from build123d import *

# Parameters (mm, degrees)
SKETCH_1_W          = 6.5
SKETCH_1_H          = 35
EXTRUDE_1_DEPTH     = 6
SKETCH_2_W          = 2.5
SKETCH_2_H          = 2.967804408
CUT_EXTRUDE_1_DEPTH = 61
SKETCH_3_W          = 6.5
SKETCH_3_H          = 15
EXTRUDE_2_DEPTH     = 4.5
SKETCH_4_W          = 6.5
SKETCH_4_H          = 1
CUT_EXTRUDE_2_DEPTH = 503.5
SKETCH_5_W          = 6.5
SKETCH_5_H          = 2
EXTRUDE_3_DEPTH     = 11.5
SKETCH_6_W          = 6.5
SKETCH_6_H          = 2
EXTRUDE_4_DEPTH     = 11.5
SKETCH_7_W          = 3.5
SKETCH_7_H          = 2.5
CUT_EXTRUDE_3_DEPTH = 90.5


with BuildPart() as part:
    # Эскиз1 → Бобышка-Вытянуть1 (new body)
    with BuildSketch(Plane(origin=(0, 0, 0), x_dir=(1, 0, 0), z_dir=(0, 1, 0))):
        with Locations((-18.856267111, 10.244186047)):
            Rectangle(SKETCH_1_W, SKETCH_1_H)
    extrude(amount=EXTRUDE_1_DEPTH)

    # Эскиз2 → Вырез-Вытянуть1 (cut)
    with BuildSketch(Plane.XY.offset(7.255813953)):
        with Locations((-18.856267111, 1.483902204)):
            Rectangle(SKETCH_2_W, SKETCH_2_H)
    extrude(amount=-CUT_EXTRUDE_1_DEPTH, mode=Mode.SUBTRACT)

    # Эскиз3 → Бобышка-Вытянуть2 (add)
    with BuildSketch(Plane(origin=(0, 6, 0), x_dir=(1, 0, 0), z_dir=(0, 1, 0))):
        with Locations((-18.856267111, 10.244186047)):
            Rectangle(SKETCH_3_W, SKETCH_3_H)
    extrude(amount=EXTRUDE_2_DEPTH)

    # Эскиз4 → Вырез-Вытянуть2 (cut)
    with BuildSketch(Plane.XY.offset(7.255813953)):
        with Locations((-18.856267111, 0.5)):
            Rectangle(SKETCH_4_W, SKETCH_4_H)
    extrude(amount=-CUT_EXTRUDE_2_DEPTH, mode=Mode.SUBTRACT)

    # Эскиз5 → Бобышка-Вытянуть3 (add)
    with BuildSketch(Plane(origin=(0, 6, 0), x_dir=(1, 0, 0), z_dir=(0, 1, 0))):
        with Locations((-18.856267111, 18.744186047)):
            Rectangle(SKETCH_5_W, SKETCH_5_H)
    extrude(amount=EXTRUDE_3_DEPTH)

    # Эскиз6 → Бобышка-Вытянуть4 (add)
    with BuildSketch(Plane(origin=(0, 6, 0), x_dir=(1, 0, 0), z_dir=(0, 1, 0))):
        with Locations((-18.856267111, 1.744186047)):
            Rectangle(SKETCH_6_W, SKETCH_6_H)
    extrude(amount=EXTRUDE_4_DEPTH)

    # Эскиз7 → Вырез-Вытянуть3 (cut)
    with BuildSketch(Plane.XY.offset(7.255813953)):
        with Locations((-18.856267111, 2.25)):
            Rectangle(SKETCH_7_W, SKETCH_7_H)
    extrude(amount=-CUT_EXTRUDE_3_DEPTH, mode=Mode.SUBTRACT)


solid = part.part
Geometry: final body of the model. Coordinates: model frame, mm. A direction names the side the tool comes from. Give positions to 0.01 mm unless a question says otherwise; leave off trailing zeros. Write each loop counter-clockwise with the first axis right and the second up, starting at its lowest first coordinate (ties: lowest second). Pieces come first, ordered by that corner, then holes. Notation, with made-up numbers: (64, 8.25) -> (86, 8.25) arc R26 cw to (86, 35.25) -> close; hole circle Ø6 at (53.25, -30). An arc over 180 degrees is marked (long way). Answer as a JSON object with one key per item and string values.
1. Cut plane D-D on y = 6.75. Output: boundary loops of the cut face in (x, z), and give its area (4 significant figures).
Ans:
{"outline": "(-22.11, -19.74) -> (-15.61, -19.74) -> (-15.61, -0.74) -> (-22.11, -0.74) -> close", "area": "123.5 mm^2"}
2. Cut plane C-C on z = 3. Output: boundary loops of the cut face in (x, y), and give its area (4 significant figures).
Ans:
{"outline": "(-22.11, 1) -> (-20.61, 1) -> (-20.61, 3.5) -> (-17.11, 3.5) -> (-17.11, 1) -> (-15.61, 1) -> (-15.61, 6) -> (-22.11, 6) -> close", "area": "23.75 mm^2"}
3. Access query for faces 1 (the flat face through (-20.606, 2, -10)), 2 (the flat face through (-19, 6, -24)), 3 (the flat face through (-19, 6, 3)). Directions: +Z, -Z, +X, -X, +Y, -Y. A direction counts if a zero-diameter tool reaches every point of the face in a straight line with its end or side. Return the directions, or none.
Ans:
{"face 1": "+Z, -Z, -Y", "face 2": "-Z, +X, -X, +Y", "face 3": "+Z, +X, -X, +Y"}
4. Mould query, pull axis Z, two halves, no side actions, for faces 4 (the flat face through (-19, 12, -0.744)), 5 (the flat face through (-19, 17.5, -19)), 6 (the flat face through (-19, 10.5, -10)), 7 (the flat face through (-19, 14, -2.744)). Classes: pulls with the +Z half, pulls with the -Z half, needs draft (parallel to the pull), parting line crosses it, or undercut.
Ans:
{"face 4": "pulls with the +Z half", "face 5": "needs draft", "face 6": "undercut", "face 7": "undercut"}
5. Cut plane B-B on x = -17.5. Output: boundary loops of the cut face in (y, z).
Ans:
{"outline": "(3.5, -27.74) -> (6, -27.74) -> (6, -19.74) -> (17.5, -19.74) -> (17.5, -17.74) -> (10.5, -17.74) -> (10.5, -2.74) -> (17.5, -2.74) -> (17.5, -0.74) -> (6, -0.74) -> (6, 7.26) -> (3.5, 7.26) -> close"}
6. Cut plane A-A on y = 14. Output: boundary loops of the cut face in (x, z), and give its area (3 significant figures).
Ans:
{"outline": "(-22.11, -19.74) -> (-15.61, -19.74) -> (-15.61, -17.74) -> (-22.11, -17.74) -> close; (-22.11, -2.74) -> (-15.61, -2.74) -> (-15.61, -0.74) -> (-22.11, -0.74) -> close", "area": "26.0 mm^2"}
7. Contact query for flat-ended pins moving along their axis: pin 1 (3 mm diameter, centred on x = -19.5, y = 15.5, fed in from +Z); pin 2 (2 mm diameter, centred on x = -19.5, z = -13, fed in from +Y); pin 3 (3 mm diameter, centred on x = -20, z = -25.5, fed in from +Y). Output: stop coordinate, or through.
Ans:
{"pin 1": "stops at z = -0.74", "pin 2": "stops at y = 10.5", "pin 3": "stops at y = 6"}
8. Ray query, probe 1 along X at (y, z) = (2.5, -11); probe 2 along Z at (x, y) = (-20.25, 11.5); probe 3 along Z at (x, y) = (-17.75, 8.25). Return the intervals inside material, ascending. Write a range as from..to.
Ans:
{"probe 1": "x = -22.11..-20.61, -17.11..-15.61", "probe 2": "z = -19.74..-17.74, -2.74..-0.74", "probe 3": "z = -19.74..-0.74"}
